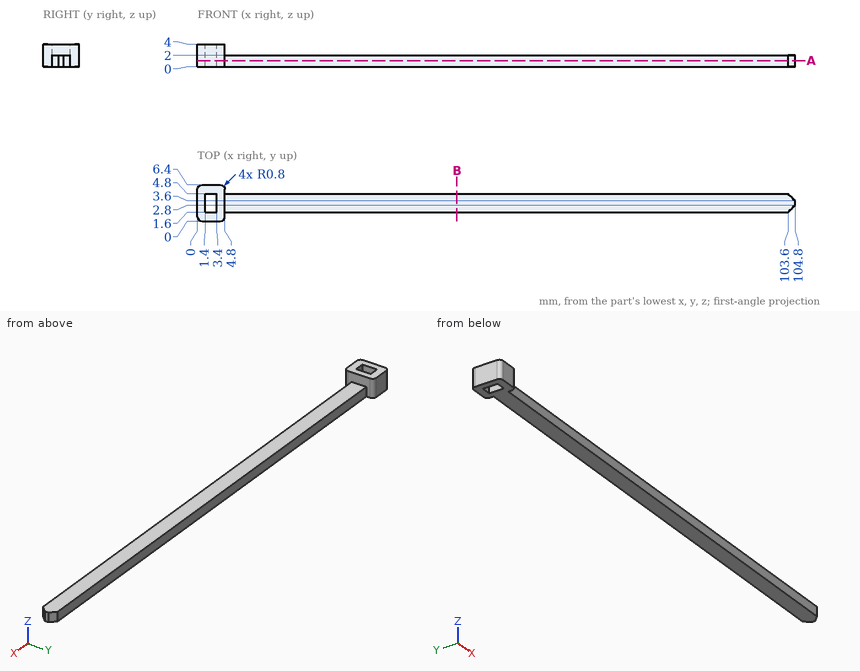
Geometry: see drawing. Coordinates: mm, zero at the bounding-box minimum. Round coordinates to 2 decimals unless told otherwise and drop trailing zeros. Order: outer loops, then holes, each group sorted by start corner. A loop starts at its lowest first (then second) coordinate and runs counter-clockwise, first axis right, second up. Notation, with made-up numbers: (27, -12) -> (64, -12) arc R31 ccw to (64, 13) -> close; hole circle Ø4 at (-26, -22). An arc over 180 degrees is marked (long way). Answer as CSV lines item,"result".
Item 1: Section A-A, the plane z = 1.1. Return loops of the section in (x, y).
A:
outline,"(0, 0.8) arc R0.8 ccw to (0.8, 0) -> (4, 0) arc R0.8 ccw to (4.8, 0.8) -> (4.8, 1.6) -> (103.6, 1.6) -> (104.8, 2.8) -> (104.8, 3.6) -> (103.6, 4.8) -> (4.8, 4.8) -> (4.8, 5.6) arc R0.8 ccw to (4, 6.4) -> (0.8, 6.4) arc R0.8 ccw to (0, 5.6) -> close; hole (1.4, 1.6) -> (3.4, 1.6) -> (3.4, 4.8) -> (1.4, 4.8) -> close"
Item 2: Section B-B, the plane x = 45.5. Return loops of the section in (y, z).
A:
outline,"(1.6, 0) -> (4.8, 0) -> (4.8, 2) -> (1.6, 2) -> close"
Item 3: Pin query (flat end, axial travel): pin 1 Ø1 at (x, z) = (81.5, 0.5) entering from +Y; pin 2 Ø0.6 at (x, z) = (33, 0.5) entering from -Y; pin 3 Ø3.5 at (x, y) = (62.5, 3.5) entering from +Z. Return the tip coordinate at first contact, or that it passes through.
A:
pin 1,"y = 4.8"
pin 2,"y = 1.6"
pin 3,"z = 2"
Item 4: Line query: L1, parallel to X at y = 3.5, z = 2.1; L2, parallel to Z at x = 35.5, y = 3.75; L3, parallel to X at y = 1, z = 1.9. Output: solid intervals per line, ascending.
A:
L1,"0 to 1.4, 3.4 to 4.8"
L2,"0 to 2"
L3,"0 to 4.8"
